The listing builds one solid part. Answer for the finished solid, in the listing's coordinates (mm). A direction names the side the tool comes from. Coordinates: 2 decimals unless noted, no trailing zeros. Order: outer loops, then holes, each group sorted by start corner. A loop starts at its lowest first (then second) coordinate and runs counter-clockwise, first axis right, second up. Notation, with made-up numbers: (23, 67.5) -> (44, 67.5) arc R20 ccw to (44, 91.5) -> close; hole circle Ø5 at (37.5, 27). An arc over 180 degrees is marked (long way). Write item = value, one per line.
from build123d import *

# Parameters (mm, degrees)
SKETCH1_R           = 1.95
SKETCH1_R_2         = 4.95
SKETCH1_R_3         = 1.5
SKETCH1_W           = 4
SKETCH1_H           = 3
SKETCH1_W_2         = 8
BOSS_EXTRUDE1_DEPTH = 3


with BuildPart() as part:
    # Sketch1 → Boss-Extrude1 (new body)
    with BuildSketch(Plane.XY):
        with BuildLine():
            Line((10.452483063, 212.041147496), (13.452483063, 212.041147496))
            Line((13.452483063, 212.041147496), (13.452483063, 209.041147496))
            Line((13.452483063, 209.041147496), (36.688713563, 209.041147496))
            Line((36.688713563, 209.041147496), (36.688713563, 212.041147496))
            Line((36.688713563, 212.041147496), (39.688713563, 212.041147496))
            Line((39.688713563, 212.041147496), (39.688713563, 209.041147496))
            Line((39.688713563, 209.041147496), (41.820598563, 209.041147496))
            Line((41.820598563, 209.041147496), (41.820598563, 162.941147496))
            Line((41.820598563, 162.941147496), (39.688713563, 162.941147496))
            Line((39.688713563, 162.941147496), (39.688713563, 159.941147496))
            Line((39.688713563, 159.941147496), (36.688713563, 159.941147496))
            Line((36.688713563, 159.941147496), (36.688713563, 162.941147496))
            Line((36.688713563, 162.941147496), (13.452483063, 162.941147496))
            Line((13.452483063, 162.941147496), (13.452483063, 159.941147496))
            Line((13.452483063, 159.941147496), (10.452483063, 159.941147496))
            Line((10.452483063, 159.941147496), (10.452483063, 162.941147496))
            Line((10.452483063, 162.941147496), (8.220599063, 162.941147496))
            Line((8.220599063, 162.941147496), (8.220599063, 165.173047496))
            Line((8.220599063, 165.173047496), (5.220599063, 165.173047496))
            Line((5.220599063, 165.173047496), (5.220599063, 168.173047496))
            Line((5.220599063, 168.173047496), (8.220599063, 168.173047496))
            Line((8.220599063, 168.173047496), (8.220599063, 197.67702847))
            ThreePointArc((8.220599063, 197.67702847), (9.220599063, 198.67702847), (8.220599063, 199.67702847))
            Line((8.220599063, 199.67702847), (8.220599063, 203.809247496))
            Line((8.220599063, 203.809247496), (5.220599063, 203.809247496))
            Line((5.220599063, 203.809247496), (5.220599063, 206.809247496))
            Line((5.220599063, 206.809247496), (8.220599063, 206.809247496))
            Line((8.220599063, 206.809247496), (8.220599063, 209.041147496))
            Line((8.220599063, 209.041147496), (10.452483063, 209.041147496))
            Line((10.452483063, 209.041147496), (10.452483063, 212.041147496))
        make_face()
        with Locations((22.320563722, 174.991147496)):
            Circle(SKETCH1_R, mode=Mode.SUBTRACT)
        with Locations((22.320563722, 196.991147496)):
            Circle(SKETCH1_R, mode=Mode.SUBTRACT)
        with Locations((22.320563664, 185.991147472)):
            Circle(SKETCH1_R_2, mode=Mode.SUBTRACT)
        with Locations((23.136540813, 202.541147496)):
            Circle(SKETCH1_R_3, mode=Mode.SUBTRACT)
        with Locations((23.136540813, 169.441147496)):
            Circle(SKETCH1_R_3, mode=Mode.SUBTRACT)
        with Locations((38.384299654, 187.07114189)):
            Circle(SKETCH1_R_3, mode=Mode.SUBTRACT)
        with BuildLine():
            Line((24.570563601, 195.140420085), (24.570563601, 191.553296454))
            ThreePointArc((24.570563601, 191.553296454), (26.563204369, 190.233788261), (27.882712601, 188.241147519))
            Line((27.882712601, 188.241147519), (31.530290537, 188.241147451))
            ThreePointArc((31.530290537, 188.241147451), (29.008711809, 192.657465398), (24.570563601, 195.140420085))
        make_face(mode=Mode.SUBTRACT)
        with BuildLine():
            Line((24.570563644, 180.428998653), (24.570563644, 176.681005512))
            ThreePointArc((24.570563644, 176.681005512), (29.067254316, 179.222501964), (31.569508813, 183.741147077))
            Line((31.569508813, 183.741147077), (27.882712476, 183.741147475))
            ThreePointArc((27.882712476, 183.741147475), (26.563204309, 181.748506814), (24.570563644, 180.428998653))
        make_face(mode=Mode.SUBTRACT)
        with BuildLine():
            Line((20.070563652, 195.14042048), (20.070563706, 191.55329637))
            ThreePointArc((20.070563706, 191.55329637), (18.077922992, 190.233788194), (16.758414793, 188.241147496))
            Line((16.758414793, 188.241147496), (13.110836488, 188.241147112))
            ThreePointArc((13.110836488, 188.241147112), (15.632415205, 192.657465481), (20.070563652, 195.14042048))
        make_face(mode=Mode.SUBTRACT)
        with BuildLine():
            Line((20.070563635, 180.428998551), (20.070563635, 176.68100541))
            ThreePointArc((20.070563635, 176.68100541), (15.573873029, 179.222501964), (13.071618593, 183.741147101))
            Line((13.071618593, 183.741147101), (16.758414722, 183.741147496))
            ThreePointArc((16.758414722, 183.741147496), (18.077922913, 181.748506761), (20.070563635, 180.428998551))
        make_face(mode=Mode.SUBTRACT)
        with Locations((15.452483063, 202.541147496)):
            Rectangle(SKETCH1_W, SKETCH1_H, mode=Mode.SUBTRACT)
        with Locations((32.820598563, 202.541147496)):
            Rectangle(SKETCH1_W_2, SKETCH1_H, mode=Mode.SUBTRACT)
        with Locations((15.452483063, 169.441147496)):
            Rectangle(SKETCH1_W, SKETCH1_H, mode=Mode.SUBTRACT)
        with Locations((32.820598563, 169.441147496)):
            Rectangle(SKETCH1_W_2, SKETCH1_H, mode=Mode.SUBTRACT)
    extrude(amount=BOSS_EXTRUDE1_DEPTH)


solid = part.part
Q1. Section A-A, the plane y = 176 is taken. Give the vertices of the cut face in (x, z), plus the area to 3 significant figures.
The answers:
outline = (8.22, 0) -> (20.65, 0) -> (20.65, 3) -> (8.22, 3) -> close; (23.99, 0) -> (41.82, 0) -> (41.82, 3) -> (23.99, 3) -> close
area = 90.8 mm2
Q2. The mould has two halves that part along X. Classify faces 1 (the face through (41.821, 186, 1)), 2 (the face through (8.221, 183, 1)), 3 (the face through (39.08, 185.74, 1.48)), 4 (the face through (9, 209.041, 1)): released by +X, released by -X, zero draft, split by the parting line, or undercut.
The answers:
face_1 = released by +X
face_2 = released by -X
face_3 = undercut
face_4 = zero draft
Q3. Find the intervals of material crossed by line 1 along Y through (x, z) = (33, 2.2); line 2 along Y through (x, z) = (7.5, 2.5); line 3 along X through (y, z) = (169, 0.8), in increasing order.
The answers:
line_1 = 162.94 to 167.94, 170.94 to 201.04, 204.04 to 209.04
line_2 = 165.17 to 168.17, 203.81 to 206.81
line_3 = 8.22 to 13.45, 17.45 to 21.7, 24.57 to 28.82, 36.82 to 41.82
Q4. A tool of negligible diameter and unlimited length cuts with its end or side. For faces 5 (the face through (41, 162.941, 1)), 6 (the face through (15, 201.041, 1)), 7 (the face through (8.221, 202, 1)), from which of +Z, -Z, +X, -X, +Y, -Y can it reach the whole face along a straight path? Write none if from no direction.
The answers:
face_5 = +Z, -Z, +X, -Y
face_6 = +Z, -Z
face_7 = +Z, -Z, -X
Q5. Section B-B, the plane x = 18.5 is taken. Give the vertices of the cut face in (y, z), plus the area to 3 significant figures.
The answers:
outline = (162.94, 0) -> (177.21, 0) -> (177.21, 3) -> (162.94, 3) -> close; (181.36, 0) -> (182.84, 0) -> (182.84, 3) -> (181.36, 3) -> close; (189.14, 0) -> (190.62, 0) -> (190.62, 3) -> (189.14, 3) -> close; (194.61, 0) -> (209.04, 0) -> (209.04, 3) -> (194.61, 3) -> close
area = 95.0 mm2
Q6. Section C-C, the plane z = 2.3 is taken. Give the number of separate pieces and of enclosed holes in the cut face, plus the area to 3 significant figures.
The answers:
separate_pieces = 1
enclosed_holes = 14
area = 1,300 mm2
Q7. Each of these flat-tipped pins is pushed along its axis until it touches: pin 1 Ø1.5 at (x, z) = (6, 1) entering from +Y; pin 2 Ø0.9 at (y, z) = (162, 1) entering from +X; pin 3 Ø0.9 at (x, z) = (14.5, 1.5) entering from +Y. Where does it stop, or does it pass through?
The answers:
pin_1 = 206.81
pin_2 = 39.69
pin_3 = 209.04
